Here's how the part is built. I have some questions about the finished solid (model axes, mm). Face numbers are marked on the shaded views. A direction names the side the tool comes from. Round coordinates to 2 decimals unless told otherwise and drop trailing zeros. Order: outer loops, then holes, each group sorted by start corner. A loop starts at its lowest first (then second) coordinate and runs counter-clockwise, first axis right, second up. Notation, with made-up numbers: (14.25, 71.25) -> (64.25, 71.25) arc R17 cw to (64.25, 90.25) -> close; hole circle Ø5 at (68, -15). An arc over 180 degrees is marked (long way). Answer in a Markdown table with one row per item.
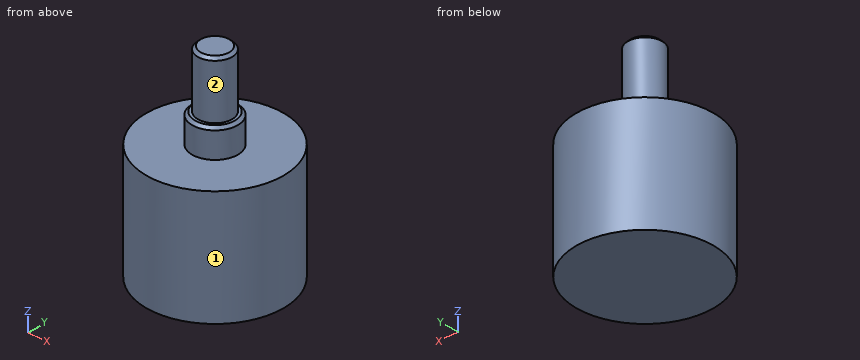
```python
from build123d import *

# Parameters (mm, degrees)
SKETCH_R     = 12
PAD_DEPTH    = 20.2
SKETCH001_R  = 3
PAD001_DEPTH = 15
SKETCH002_R  = 4
PAD002_DEPTH = 5
CHAMFER_SIZE = 0.5


with BuildPart() as part:
    # Sketch → Pad (new body)
    with BuildSketch(Plane.XY):
        Circle(SKETCH_R)
    extrude(amount=-PAD_DEPTH)

    # Sketch001 → Pad001 (join)
    with BuildSketch(Plane.XY):
        Circle(SKETCH001_R)
    extrude(amount=PAD001_DEPTH)

    # Sketch002 → Pad002 (join)
    with BuildSketch(Plane.XY):
        Circle(SKETCH002_R)
    extrude(amount=PAD002_DEPTH)

    # Chamfer
    chamfer_edges = [part.edges().sort_by_distance(p)[0] for p in [
        (-4, 0, 5),
        (-3, 0, 15),
    ]]
    chamfer(chamfer_edges, length=CHAMFER_SIZE)


solid = part.part
```
1. Suppose I cut it at A-A on x = 0. Write out the boundary of the cut face in (y, z).
Numbers:
| item | result |
|---|---|
| outline | (-12, -20.2) -> (12, -20.2) -> (12, 0) -> (4, 0) -> (4, 4.5) -> (3.5, 5) -> (3, 5) -> (3, 14.5) -> (2.5, 15) -> (-2.5, 15) -> (-3, 14.5) -> (-3, 5) -> (-3.5, 5) -> (-4, 4.5) -> (-4, 0) -> (-12, 0) -> close |
2. Please list where these lines run through material, in increasing order: line 1 along Z through (x, y) = (7, 8.5); line 2 along X through (y, z) = (-1, 8.5); line 3 along X through (y, z) = (1, -5.5).
Numbers:
| item | result |
|---|---|
| line 1 | z = -20.2 to 0 |
| line 2 | x = -2.83 to 2.83 |
| line 3 | x = -11.96 to 11.96 |
3. For the marked faces 1 and 2, which set-ups out of +Z, -Z, +X, -X, +Y, -Y let a thin tool reach every point of the face, with its end or its side?
Numbers:
| item | result |
|---|---|
| face 1 | +Z, -Z |
| face 2 | +Z |
4. Suppose I cut it at D-D on z = -15.5. Write out the boundary of the cut face in (x, y).
Numbers:
| item | result |
|---|---|
| outline | circle Ø24 at (0, 0) |
5. Suppose I cut it at C-C on z = 3. Write out the boundary of the cut face in (x, y).
Numbers:
| item | result |
|---|---|
| outline | circle Ø8 at (0, 0) |
6. For pin 1 Ø1 at (x, z) = (7.5, -10) entering from -Y; pin 2 Ø10 at (x, z) = (4.5, 3.5) entering from +Y; pin 3 Ø4 at (x, z) = (5, -6.5) entering from -Y, each with a flat end and sliding along its axis, tell me the tip position at first contact or that it passes through.
Numbers:
| item | result |
|---|---|
| pin 1 | stops at y = -9.75 |
| pin 2 | stops at y = 11.96 |
| pin 3 | stops at y = -11.62 |
